Geometry: see drawing. Coordinates: mm, zero at the bounding-box minimum. A direction names the side the tool comes from. Round coordinates to 2 decimals unless told otherwise and drop trailing zeros. Loops run counter-clockwise (first coordinate to the right, second up) from the corner with the lowest first, then second, coordinate; pieces in that order, holes last.
(1) Section A-A, the plane z = 7.5. Return the cut outline in (x, y), plus the area to 3 significant figures.
(2) Section C-C, the plane z = 15. Return the cut outline in (x, y), plus the area to 3 significant figures.
(3) Section D-D, the plane x = 46.5. Return the cut outline in (y, z).
(4) Set-up query: the marked faces 1, 2, 3 and 4. Return all of +Z, -Z, +X, -X, +Y, -Y with unobstructed straight access to the full face (end or side cutting, diameter ignored); none if empty.
(5) Material intervals for probe 1 along X at (y, z) = (69, 13.5); probe 2 along X at (y, z) = (36.5, 10); probe 3 along X at (y, z) = (64, 21.5), sorted ascending.
(6) First-contact query: pin 1 Ø2 at (y, z) = (55, 21.5) entering from -X; pin 2 Ø15 at (y, z) = (48, 12) entering from +X; pin 3 Ø7.5 at (x, y) = (6.5, 56) entering from +Z. Flat tips, straight axial feed; report the tip coordinate or a pass-through.
(7) Section B-B, the plane y = 71.5. Return the cut outline in (x, z), plus the area to 3 significant figures.
(8) Mould query, pull axis X, two halves, no side actions, for the marked faces 5, 6 and 7. Classes: pulls with the +X half, pulls with the -X half, needs draft (parallel to the pull), parting line crosses it, or undercut.
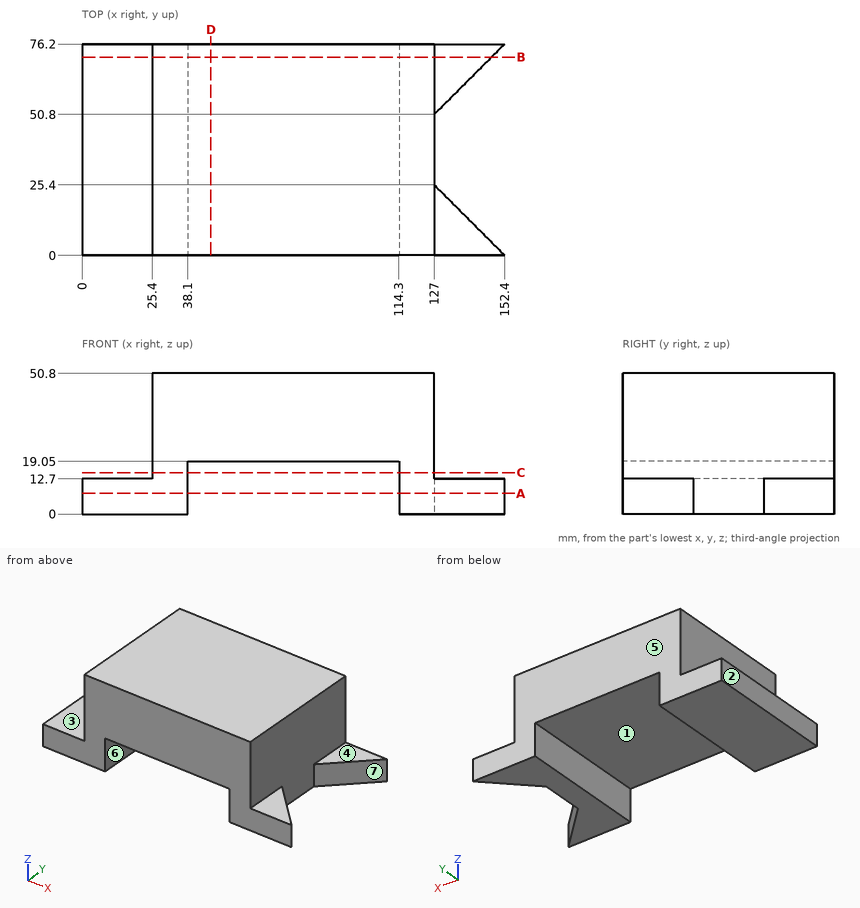
Output values:
1. outline: (0, 0) - (38.1, 0) - (38.1, 76.2) - (0, 76.2) - close; (114.3, 0) - (152.4, 0) - (127, 25.4) - (127, 50.8) - (152.4, 76.2) - (114.3, 76.2) - close
1. area: 4,520 mm2
2. outline: (25.4, 0) - (38.1, 0) - (38.1, 76.2) - (25.4, 76.2) - close; (114.3, 0) - (127, 0) - (127, 76.2) - (114.3, 76.2) - close
2. area: 1,940 mm2
3. outline: (0, 19.05) - (76.2, 19.05) - (76.2, 50.8) - (0, 50.8) - close
4. face 1: -Z, +Y, -Y
4. face 2: +Z, -Z, -X, +Y, -Y
4. face 3: +Z, -X, +Y, -Y
4. face 4: +Z, +X, +Y, -Y
5. probe 1: x = 25.4 to 38.1, 114.3 to 127
5. probe 2: x = 0 to 38.1, 114.3 to 127
5. probe 3: x = 25.4 to 127
6. pin 1: stops at x = 25.4
6. pin 2: stops at x = 131.7
6. pin 3: stops at z = 12.7
7. outline: (0, 0) - (38.1, 0) - (38.1, 19.05) - (114.3, 19.05) - (114.3, 0) - (147.7, 0) - (147.7, 12.7) - (127, 12.7) - (127, 50.8) - (25.4, 50.8) - (25.4, 12.7) - (0, 12.7) - close
7. area: 4,300 mm2
8. face 5: needs draft
8. face 6: undercut
8. face 7: pulls with the +X half
